Part model, mm, in its own coordinate system. A direction names the side the tool comes from. Round coordinates to 2 decimals unless told otherwise and drop trailing zeros. Write each loop counter-clockwise with the first axis right and the second up, starting at its lowest first coordinate (ties: lowest second). Pieces come first, ordered by that corner, then holes.
from build123d import *

# Parameters (mm, degrees)
BOSS_EXTRUDE1_DEPTH   = 2.54
F_8_CLEARANCE_HOLE1_D = 4.9149


with BuildPart() as part:
    # Sketch1 → Boss-Extrude1 (new body)
    with BuildSketch(Plane.XY):
        with BuildLine():
            Line((258.7625, 71.196211277), (249.2375, 71.196211277))
            ThreePointArc((249.2375, 71.196211277), (244.747371939, 73.056083217), (242.8875, 77.546211277))
            Line((242.8875, 77.546211277), (242.8875, 101.893951031))
            ThreePointArc((242.8875, 101.893951031), (240.954040126, 111.614110214), (235.448012242, 119.854463274))
            Line((235.448012242, 119.854463274), (192.383237758, 162.919237758))
            ThreePointArc((192.383237758, 162.919237758), (136.442161509, 200.297869889), (70.455162895, 213.4235))
            Line((70.455162895, 213.4235), (-70.455162895, 213.4235))
            ThreePointArc((-70.455162895, 213.4235), (-136.442161509, 200.297869889), (-192.383237758, 162.919237758))
            Line((-192.383237758, 162.919237758), (-235.448012242, 119.854463274))
            ThreePointArc((-235.448012242, 119.854463274), (-240.954040126, 111.614110214), (-242.8875, 101.893951031))
            Line((-242.8875, 101.893951031), (-242.8875, 77.546211277))
            ThreePointArc((-242.8875, 77.546211277), (-244.747371939, 73.056083217), (-249.2375, 71.196211277))
            Line((-249.2375, 71.196211277), (-258.7625, 71.196211277))
            ThreePointArc((-258.7625, 71.196211277), (-263.252628061, 73.056083217), (-265.1125, 77.546211277))
            Line((-265.1125, 77.546211277), (-265.1125, 115.589975516))
            ThreePointArc((-265.1125, 115.589975516), (-263.179040126, 125.310134698), (-257.673012242, 133.550487758))
            Line((-257.673012242, 133.550487758), (-148.726987758, 242.496512242))
            ThreePointArc((-148.726987758, 242.496512242), (-140.486634698, 248.002540126), (-130.766475516, 249.936))
            Line((-130.766475516, 249.936), (130.766475516, 249.936))
            ThreePointArc((130.766475516, 249.936), (140.486634698, 248.002540126), (148.726987758, 242.496512242))
            Line((148.726987758, 242.496512242), (257.673012242, 133.550487758))
            ThreePointArc((257.673012242, 133.550487758), (263.179040126, 125.310134698), (265.1125, 115.589975516))
            Line((265.1125, 115.589975516), (265.1125, 77.546211277))
            ThreePointArc((265.1125, 77.546211277), (263.252628061, 73.056083217), (258.7625, 71.196211277))
        make_face()
    extrude(amount=BOSS_EXTRUDE1_DEPTH)

    # #8 Clearance Hole1 (through all)
    with Locations(Plane(origin=(0, 0, 0), x_dir=(-1, 0, 0), z_dir=(0, 0, -1))):
        with Locations((-254, 88.9635), (-252.044186638, 121.21880112), (-234.083674396, 139.179313362), (-216.123162153, 157.139825604), (-198.162649911, 175.100337847), (-180.202137669, 193.060850089), (-114.3, 238.8235), (-88.9, 238.8235), (-63.5, 238.8235), (-38.1, 238.8235), (-12.7, 238.8235), (12.7, 238.8235), (38.1, 238.8235), (63.5, 238.8235), (88.9, 238.8235), (114.3, 238.8235), (139.7, 238.8235), (162.241625427, 211.021362331), (180.202137669, 193.060850089), (198.162649911, 175.100337847), (216.123162153, 157.139825604), (234.083674396, 139.179313362), (252.044186638, 121.21880112), (254, 88.9635), (-139.7, 238.8235), (-162.241625427, 211.021362331)):
            Hole(F_8_CLEARANCE_HOLE1_D / 2)


solid = part.part
Q1. Saw through at B-B, the plane x = 25. Write the cut outline in (y, z).
Q2. Drop flat-ended pins along their axis: P1, Ø1.5, axis at y = 197, z = 1.5, coming from the -X side; P2, Ø4, axis at x = -12.7, y = 238.82, coming from the -Z side; P3, Ø1, axis at x = 29, z = 2, coming from the -Y side. Give the stop position or say it passes through.
Q3. Tool access for faces 5 (the flat face through (1, 221, 2.54)), 6 (the cylindrical face through (-135.565, 200.658, 1.252)): list every direction of +Z, -Z, +X, -X, +Y, -Y with a clear straight run to the whole face (end or side of a thin tool).
Q4. Saw through at C-C, the plane z = 2.15. Give the number of separate pieces and of enclosed holes in the cut face, and give its area (3 significant figures).
Q5. Two-plate mould, pull along X, no slides. Class faces 1 (the flat face through (-213.6, 141.7, 1.3)), 2 (the flat face through (1, 221, 0)), 3 (the cylindrical face through (137.32, 199.93, 1.25)), 4 (the flat face through (202.437, 188.786, 1.252)): released by +X, released by -X, zero draft, split by the parting line, or undercut.
Q6. Saw through at A-A, the plane y = 147. Write the cut outline in (x, z).
Q7. Wall check: line 1 (X direction, y = 119.5, z = 0.85); line 2 (X direction, y = 97.5, z = 1.2); line 3 (X direction, y = 90.5, z = 1.55). Give the ranges that are in metal, low to high.
Computed:
1. outline: (213.42, 0) - (249.94, 0) - (249.94, 2.54) - (213.42, 2.54) - close
2. P1: stops at x = -194.97
2. P2: passes through
2. P3: stops at y = 213.42
3. face 5: +Z, +X, -X, +Y, -Y
3. face 6: +Z, -Z, -Y
4. separate pieces: 1
4. enclosed holes: 26
4. area: 21,300 mm2
5. face 1: undercut
5. face 2: zero draft
5. face 3: undercut
5. face 4: released by +X
6. outline: (-244.22, 0) - (-208.3, 0) - (-208.3, 2.54) - (-244.22, 2.54) - close; (208.3, 0) - (244.22, 0) - (244.22, 2.54) - (208.3, 2.54) - close
7. line 1: x = -264.81 to -253.8, -250.29 to -235.8, 235.8 to 250.29, 253.8 to 264.81
7. line 2: x = -265.11 to -242.89, 242.89 to 265.11
7. line 3: x = -265.11 to -255.92, -252.08 to -242.89, 242.89 to 252.08, 255.92 to 265.11
